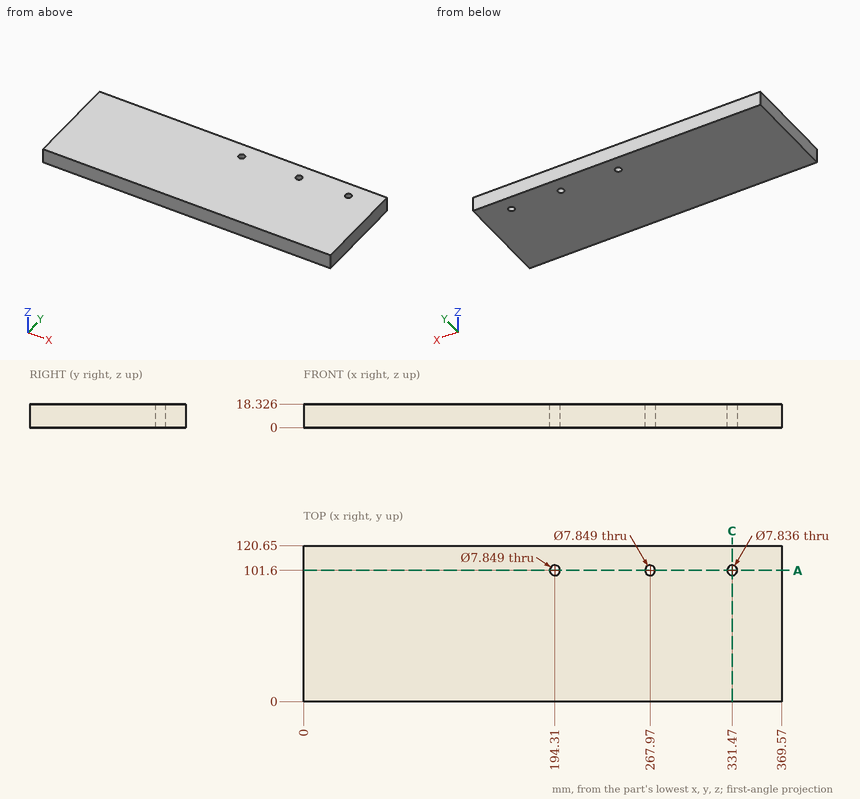
The drawing under review shows one solid part. Ordinate dimensions are in mm from its lowest x, y, z. Round coordinates to 2 decimals unless told otherwise and drop trailing zeros. Order: outer loops, then holes, each group sorted by start corner. A loop starts at its lowest first (then second) coordinate and runs counter-clockwise, first axis right, second up. Notation, with made-up numbers: (49, 8.5) -> (53, 8.5) arc R17 cw to (53, 24.5) -> close; hole circle Ø11 at (85.5, 37.25). An arc over 180 degrees is marked (long way). Use a Markdown table: item, result.
Q1. Clearance check with flat-ended pins moving along their axes: P1, Ø9, axis at x = 331.47, y = 101.6, coming from the +Z side; P2, Ø4.5, axis at x = 267.97, y = 101.6, coming from the -Z side. State where each tip first meets the part, or that it passes through.
Values:
| item | result |
|---|---|
| P1 | stops at z = 18.33 |
| P2 | passes through |
Q2. We need section A-A on y = 101.6. Write out the cut boundary in (x, z) (1 decimal), then the cut area to 3 significant figures.
Values:
| item | result |
|---|---|
| outline | (0, 0) -> (190.4, 0) -> (190.4, 18.3) -> (0, 18.3) -> close; (198.2, 0) -> (264, 0) -> (264, 18.3) -> (198.2, 18.3) -> close; (271.9, 0) -> (327.6, 0) -> (327.6, 18.3) -> (271.9, 18.3) -> close; (335.4, 0) -> (369.6, 0) -> (369.6, 18.3) -> (335.4, 18.3) -> close |
| area | 6,340 mm^2 |
Q3. We need section C-C on x = 331.47. Write out the cut boundary in (y, z).
Values:
| item | result |
|---|---|
| outline | (0, 0) -> (97.68, 0) -> (97.68, 18.33) -> (0, 18.33) -> close; (105.52, 0) -> (120.65, 0) -> (120.65, 18.33) -> (105.52, 18.33) -> close |
Q4. For line 1 (Y direction, x = 331.47, z = 10); line 2 (X direction, y = 104.5, z = 7.25) (1 decimal); line 3 (Y direction, x = 192, z = 16.75), list the stretches that pass through material, from the lowest coordinate up.
Values:
| item | result |
|---|---|
| line 1 | y = 0 to 97.68, 105.52 to 120.65 |
| line 2 | x = 0 to 191.7, 197 to 265.3, 270.6 to 328.8, 334.1 to 369.6 |
| line 3 | y = 0 to 98.43, 104.77 to 120.65 |
